Verification items for the finished model (mm, model axes). A direction names the side the tool comes from. Coordinates: 2 decimals unless noted, no trailing zeros. Write item = value, one per line. Start each with the question number.
(1) Material ranges on probe 1 along X at (y, z) = (0, 5.5); probe 2 along Y at (x, z) = (0, 7.75); probe 3 along Y at (x, z) = (15.5, 1), recorded low to high. Write a range as [from, to].
(2) Set-up check for faces 1 (the face through (-0.3, -6.2, -4.5)), 2 (the face through (0, -15, 10)), 3 (the face through (-16.296, -9.441, 21.232)), 4 (the face through (-4, -2, -0.5)): record each of +Z, -Z, +X, -X, +Y, -Y from which the full face is reachable in a straight line by a thin tool's end or side.
(3) Gauge pin test, flat ends, axial feed: pin 1 Ø2.5 at (x, y) = (-5.2, -3) entering from +Z; pin 2 Ø4 at (x, z) = (4.5, 13) entering from +Y; pin 3 Ø4 at (x, z) = (9, 14) entering from -Y. Record the tip position at first contact, or that the pin passes through.
(4) Section check A-A (x = 0). State how many separate pieces and enclosed holes the cut face has, plus the area to 3 significant figures.
(5) Mould release check, pull along Z, two halves, no side actions. Record for faces 5 (the face through (-17.5, 17.5, 1.2)), 6 (the face through (13.17, 20.66, 11.11)), 7 (the face through (5.165, 3.053, -6.226)), 8 (the face through (-12.3, 6.6, 20)): released by +Z, released by -Z, zero draft, split by the parting line, or undercut.
```python
from build123d import *
from build123d.topology import SkipClean

# Parameters (mm, degrees)
BOSS_EXTRUDE1_DEPTH      = 22.5
BOSS_EXTRUDE1_DEPTH_BACK = 0.0001
SKETCH1_R                = 24.5
SKETCH1_R_2              = 23
SKETCH4_R                = 26
SKETCH4_R_2              = 23
BOSS_EXTRUDE2_DEPTH      = 1.2
BOSS_EXTRUDE4_START      = -1.2
SKETCH7_R                = 26
SKETCH7_R_2              = 24.253874055
BOSS_EXTRUDE4_DEPTH      = 1.2
SKETCH8_R                = 15
SKETCH8_R_2              = 13.8
BOSS_EXTRUDE5_DEPTH      = 20
SKETCH9_R                = 10
BOSS_EXTRUDE6_DEPTH      = 1
SKETCH11_W               = 4
SKETCH11_H               = 2.5
BOSS_EXTRUDE8_DEPTH      = 24
SKETCH19_W               = 4
SKETCH19_H               = 9.350394366
BOSS_EXTRUDE9_DEPTH      = 20
SKETCH13_R               = 4.65
CUT_EXTRUDE7_DEPTH       = 1.5
CIRPATTERN2_COUNT        = 3
SKETCH21_R               = 4.65
CUT_EXTRUDE8_DEPTH       = 1.5
CIRPATTERN6_COUNT        = 3
SKETCH23_R               = 1.1
CUT_EXTRUDE9_DEPTH       = 3.5
CIRPATTERN8_COUNT        = 3
CUT_EXTRUDE11_DEPTH      = 4
CIRPATTERN9_COUNT        = 3
BOSS_EXTRUDE10_START     = 4
SKETCH27_R               = 10
BOSS_EXTRUDE10_DEPTH     = 4
SKETCH29_R               = 6
BOSS_EXTRUDE11_DEPTH     = 4
CUT_EXTRUDE12_START      = -13
SKETCH30_R               = 1.1
CUT_EXTRUDE12_DEPTH      = 13
CUT_EXTRUDE13_START      = -13
SKETCH31_R               = 1.1
CUT_EXTRUDE13_DEPTH      = 13
SKETCH32_R               = 1.9
CUT_EXTRUDE14_DEPTH      = 7.5
CUT_EXTRUDE15_DEPTH      = 2.5
SKETCH36_R               = 1.6
CUT_EXTRUDE16_DEPTH      = 18.5
SKETCH40_R               = 7.25
BOSS_EXTRUDE13_DEPTH     = 0.5
SKETCH36_4_R             = 1.6
CUT_EXTRUDE17_DEPTH      = 8.5
SKETCH32_3_R             = 1.9
CUT_EXTRUDE18_DEPTH      = 4.5
CIRPATTERN10_COUNT       = 3


with BuildPart() as part:
    # Sketch1 → Boss-Extrude1 (new, two sides: drawn at the far end of the back side and taken through both)
    with BuildSketch(Plane.XY.offset(-BOSS_EXTRUDE1_DEPTH_BACK)):
        Circle(SKETCH1_R)
        Circle(SKETCH1_R_2, mode=Mode.SUBTRACT)
    extrude(amount=BOSS_EXTRUDE1_DEPTH + BOSS_EXTRUDE1_DEPTH_BACK)

    # Sketch4 → Boss-Extrude2 (add)
    with SkipClean():  # the faces are left unmerged after this step: merging them gives an invalid solid
        with BuildSketch(Plane.XY):
            Circle(SKETCH4_R)
            Circle(SKETCH4_R_2, mode=Mode.SUBTRACT)
        extrude(amount=BOSS_EXTRUDE2_DEPTH)

    # Sketch7 → Boss-Extrude4 (add)
    with SkipClean():  # the faces are left unmerged after this step: merging them gives an invalid solid
        with BuildSketch(Plane.XY.offset(22.5).offset(BOSS_EXTRUDE4_START)):
            Circle(SKETCH7_R)
            with Locations((-0.246125945, 0)):
                Circle(SKETCH7_R_2, mode=Mode.SUBTRACT)
        extrude(amount=BOSS_EXTRUDE4_DEPTH)



with BuildPart() as body_2:
    # Sketch8 → Boss-Extrude5 (new body)
    with BuildSketch(Plane.XY):
        Circle(SKETCH8_R)
        Circle(SKETCH8_R_2, mode=Mode.SUBTRACT)
    extrude(amount=BOSS_EXTRUDE5_DEPTH)


with BuildPart() as body_3:
    # Sketch9 → Boss-Extrude6 (new body)
    with BuildSketch(Plane.XY):
        Circle(SKETCH9_R)
    extrude(amount=BOSS_EXTRUDE6_DEPTH)


with BuildPart() as part_1:
    add(part.part)

    add(body_2.part)  # Boss-Extrude8 merges body 2

    add(body_3.part)  # Boss-Extrude8 merges body 3
    # Sketch11 → Boss-Extrude8 (add)
    with BuildSketch(Plane(origin=(0, 0, 0), x_dir=(1, 0, 0), z_dir=(0, 1, 0))):
        with Locations((0, -1.25)):
            Rectangle(SKETCH11_W, SKETCH11_H)
    boss_extrude8 = extrude(amount=BOSS_EXTRUDE8_DEPTH)

    # Sketch19 → Boss-Extrude9 (add, through all)
    with BuildSketch(Plane.XY.offset(2.5)):
        with Locations((0, 19.250315011)):
            Rectangle(SKETCH19_W, SKETCH19_H)
    boss_extrude9 = extrude(amount=BOSS_EXTRUDE9_DEPTH)

    # Sketch13 → Cut-Extrude7 (cut)
    with BuildSketch(Plane.XY.offset(2.5)):
        Circle(SKETCH13_R)
    extrude(amount=-CUT_EXTRUDE7_DEPTH, mode=Mode.SUBTRACT)

    # CirPattern2: Boss-Extrude8 ×3 about axis
    cirpattern2_axis = Axis((0, 0, 0), (0, 0, 1))
    for i in range(1, CIRPATTERN2_COUNT):
        add(boss_extrude8.rotate(cirpattern2_axis, i * 360 / CIRPATTERN2_COUNT))

    # Sketch21 → Cut-Extrude8 (cut)
    with BuildSketch(Plane.XY.offset(2.5)):
        Circle(SKETCH21_R)
    extrude(amount=-CUT_EXTRUDE8_DEPTH, mode=Mode.SUBTRACT)

    # CirPattern6: Boss-Extrude9 ×3 about axis
    cirpattern6_axis = Axis((0, 0, 0), (0, 0, 1))
    for i in range(1, CIRPATTERN6_COUNT):
        add(boss_extrude9.rotate(cirpattern6_axis, i * 360 / CIRPATTERN6_COUNT))

    # Sketch23 → Cut-Extrude9 (cut)
    with BuildSketch(Plane(origin=(0, 0, 0), x_dir=(-1, 0, 0), z_dir=(0, 0, -1))):
        with Locations((0, 6)):
            Circle(SKETCH23_R)
    cut_extrude9 = extrude(amount=-CUT_EXTRUDE9_DEPTH, mode=Mode.SUBTRACT)

    # CirPattern8: Cut-Extrude9 ×3 about axis
    cirpattern8_axis = Axis((0, 0, 0), (0, 0, 1))
    for i in range(1, CIRPATTERN8_COUNT):
        add(cut_extrude9.rotate(cirpattern8_axis, i * 360 / CIRPATTERN8_COUNT), mode=Mode.SUBTRACT)

    # Sketch20 → Cut-Extrude11 (cut)
    with BuildSketch(Plane.ZY.offset(2)):
        Polygon((20, 14.866068747), (22.5, 22.912878475), (22.5, 14.575117828), (20, 14.575117828), align=None)
    cut_extrude11 = extrude(amount=-CUT_EXTRUDE11_DEPTH, mode=Mode.SUBTRACT)

    # CirPattern9: Cut-Extrude11 ×3 about axis
    cirpattern9_axis = Axis((0, 0, 0), (0, 0, 1))
    for i in range(1, CIRPATTERN9_COUNT):
        add(cut_extrude11.rotate(cirpattern9_axis, i * 360 / CIRPATTERN9_COUNT), mode=Mode.SUBTRACT)

    # Sketch27 → Boss-Extrude10 (add)
    with BuildSketch(Plane(origin=(0, 0, 0), x_dir=(-1, 0, 0), z_dir=(0, 0, -1)).offset(BOSS_EXTRUDE10_START)):
        Circle(SKETCH27_R)
    extrude(amount=-BOSS_EXTRUDE10_DEPTH)

    # Sketch29 → Boss-Extrude11 (add)
    with BuildSketch(Plane(origin=(0, 0, -4), x_dir=(-1, 0, 0), z_dir=(0, 0, -1))):
        Circle(SKETCH29_R)
    extrude(amount=BOSS_EXTRUDE11_DEPTH)

    # Sketch30 → Cut-Extrude12 (cut)
    with BuildSketch(Plane.XY.offset(1).offset(CUT_EXTRUDE12_START)):
        with Locations(Location((0, 6, 0), (0, 0, 180))):
            Circle(SKETCH30_R)
    extrude(amount=CUT_EXTRUDE12_DEPTH, mode=Mode.SUBTRACT)

    # Sketch31 → Cut-Extrude13 (cut)
    with BuildSketch(Plane.XY.offset(1).offset(CUT_EXTRUDE13_START)):
        with Locations(Location((5.196152423, -3, 0), (0, 0, 180))):
            Circle(SKETCH31_R)
        with Locations(Location((-5.196152423, -3, 0), (0, 0, 180))):
            Circle(SKETCH31_R)
    extrude(amount=CUT_EXTRUDE13_DEPTH, mode=Mode.SUBTRACT)

    # Sketch32 → Cut-Extrude14 (cut)
    with SkipClean():  # the faces are left unmerged after this step: merging them gives an invalid solid
        with BuildSketch(Plane(origin=(0, 0, -8), x_dir=(-1, 0, 0), z_dir=(0, 0, -1))):
            with Locations((0, 6)):
                Circle(SKETCH32_R)
        cut_extrude14 = extrude(amount=-CUT_EXTRUDE14_DEPTH, mode=Mode.SUBTRACT)
    add(part_1.part.scale(1), mode=Mode.REPLACE)  # the faces are merged on a copy

    # Sketch35 → Cut-Extrude15 (cut)
    with BuildSketch(Plane.XY.offset(1)):
        Polygon((1.58771324, -2.75), (3.175426481, 0), (1.58771324, 2.75), (-1.58771324, 2.75), (-3.175426481, 0), (-1.58771324, -2.75), align=None)
    extrude(amount=-CUT_EXTRUDE15_DEPTH, mode=Mode.SUBTRACT)

    # Sketch36 → Cut-Extrude16 (cut)
    with BuildSketch(Plane(origin=(0, 0, -8), x_dir=(-1, 0, 0), z_dir=(0, 0, -1))):
        Circle(SKETCH36_R)
    extrude(amount=-CUT_EXTRUDE16_DEPTH, mode=Mode.SUBTRACT)

    # Sketch40 → Boss-Extrude13 (add)
    with BuildSketch(Plane(origin=(0, 0, -4), x_dir=(-1, 0, 0), z_dir=(0, 0, -1))):
        with Locations(Location((0, 0, 0), (0, 0, 102.455047825))):
            Circle(SKETCH40_R)
    extrude(amount=BOSS_EXTRUDE13_DEPTH)

    # Sketch36<4> → Cut-Extrude17 (cut)
    with BuildSketch(Plane(origin=(0, 0, -8), x_dir=(-1, 0, 0), z_dir=(0, 0, -1))):
        Circle(SKETCH36_4_R)
    extrude(amount=-CUT_EXTRUDE17_DEPTH, mode=Mode.SUBTRACT)

    # Sketch32<3> → Cut-Extrude18 (cut)
    with BuildSketch(Plane(origin=(0, 0, -8), x_dir=(-1, 0, 0), z_dir=(0, 0, -1))):
        with Locations((0, 6)):
            Circle(SKETCH32_3_R)
    extrude(amount=-CUT_EXTRUDE18_DEPTH, mode=Mode.SUBTRACT)

    # CirPattern10: Cut-Extrude14 ×3 about axis
    cirpattern10_axis = Axis((0, 0, 0), (0, 0, 1))
    for i in range(1, CIRPATTERN10_COUNT):
        add(cut_extrude14.rotate(cirpattern10_axis, i * 360 / CIRPATTERN10_COUNT), mode=Mode.SUBTRACT)


solid = part_1.part
```
Response:
q1.probe_1 = [-24.5, -23], [-15, -13.8], [13.8, 15], [23, 24.5]
q1.probe_2 = [-24.5, -23], [-15, -13.8], [13.8, 24.5]
q1.probe_3 = [-20.87, -16.99], [-11.26, -6.64], [16.99, 20.87]
q2.face_1 = -Z, -Y
q2.face_2 = +Z, -Z
q2.face_3 = +Z
q2.face_4 = -Z
q3.pin_1 = 2.5
q3.pin_2 = 24.37
q3.pin_3 = -23.48
q4.separate_pieces = 5
q4.enclosed_holes = 0
q4.area = 397 mm2
q5.face_5 = undercut
q5.face_6 = undercut
q5.face_7 = zero draft
q5.face_8 = released by +Z
